Here's how the part is built. I have some questions about the finished solid (model axes, mm). A direction names the side the tool comes from. Round coordinates to 2 decimals unless told otherwise and drop trailing zeros. Write each loop counter-clockwise with the first axis right and the second up, starting at its lowest first coordinate (ties: lowest second). Pieces come first, ordered by that corner, then holes. Notation, with made-up numbers: (70, -21.5) -> (76, -21.5) arc R37 ccw to (76, 14.5) -> close; hole circle Ø2 at (8.5, 54). An arc over 180 degrees is marked (long way). Put each result on its own line as item: value. Start each with the question number.
1. I need wall thicknesses on probe 1 along X at (y, z) = (-10, 26); probe 2 along Z at (x, y) = (2.5, 9); probe 3 along Y at (x, z) = (-11, 14). Which ranges of each line are inside material? Lowest first, please. Write a range as from..to.
2. Suppose I cut it at D-D (y = 4). Please give me the cut outline in (x, z).
3. Suppose I cut it at C-C (z = 18). Please give me the cut outline in (x, y).
4. For pin 1 (8.5 mm diameter, centred on y = -4, z = 9, fed in from +X); pin 2 (5 mm diameter, centred on x = -23.5, z = 14.5, fed in from +Y); pin 3 (10 mm diameter, centred on x = -1, y = 12, fed in from +Z), each with a flat end and sliding along its axis, tell me the tip position at first contact or that it passes through.
5. Which directions (+Z, -Z, +X, -X, +Y, -Y) give clear straight access to the entire face, cutting with the end or side of a thin tool? Please do faces 1 (the face through (-6, 7, 0)), 2 (the face through (-10, 2, -20)), 3 (the face through (-10, -10, 15)), 4 (the face through (-20, -14, 30)), 5 (the face through (-20, 0, 15)).
6. Suppose I cut it at A-A (x = -11.5). Please give me the cut outline in (y, z), then the cut area to 3 significant figures.
7. Suppose I cut it at B-B (y = -14). Please give me the cut outline in (x, z), then the cut area to 3 significant figures.
```python
from build123d import *

# Parameters (mm, degrees)
SKETCH1_W           = 20
SKETCH1_H           = 18
BOSS_EXTRUDE1_DEPTH = 30
SKETCH2_W           = 40
SKETCH2_H           = 40
BOSS_EXTRUDE2_DEPTH = 20
FILLET1_R           = 10


with BuildPart() as part:
    # Sketch1 → Boss-Extrude1 (new body)
    with BuildSketch(Plane.XY):
        with Locations((-20, -9)):
            Rectangle(SKETCH1_W, SKETCH1_H)
    extrude(amount=BOSS_EXTRUDE1_DEPTH)

    # Sketch2 → Boss-Extrude2 (add)
    with BuildSketch(Plane.XY):
        with Locations((-10, 2)):
            Rectangle(SKETCH2_W, SKETCH2_H)
    extrude(amount=-BOSS_EXTRUDE2_DEPTH)

    # Fillet1
    fillet1_edges = [part.edges().sort_by_distance(p)[0] for p in [
        (10, 22, -10),
        (-20, 0, 30),
        (-20, 0, 0),
    ]]
    fillet(fillet1_edges, radius=FILLET1_R)


solid = part.part
```
Verdict:
1. probe 1: x = -30..-10
1. probe 2: z = -20..0
1. probe 3: y = -18..0
2. outline: (-30, -20) -> (10, -20) -> (10, 0) -> (-10, 0) -> (-10, 2) -> (-30, 2) -> close
3. outline: (-30, -18) -> (-10, -18) -> (-10, 0) -> (-30, 0) -> close
4. pin 1: stops at x = -10
4. pin 2: stops at y = 0
4. pin 3: stops at z = 0
5. face 1: +Z, +X, +Y
5. face 2: -Z, +X, -X, +Y, -Y
5. face 3: +Z, +X, +Y, -Y
5. face 4: +Z, +X, -X, +Y, -Y
5. face 5: +Z, +X, -X, +Y
6. outline: (-18, -20) -> (22, -20) -> (22, 0) -> (10, 0) arc R10 cw to (0, 10) -> (0, 20) arc R10 ccw to (-10, 30) -> (-18, 30) -> close
6. area: 1,340 mm^2
7. outline: (-30, -20) -> (10, -20) -> (10, 0) -> (-10, 0) -> (-10, 30) -> (-30, 30) -> close
7. area: 1,400 mm^2
